Design review of the part built by this model. Coordinates are the model's own, in mm. Coordinates: 2 decimals unless noted, no trailing zeros. Order: outer loops, then holes, each group sorted by start corner. A loop starts at its lowest first (then second) coordinate and runs counter-clockwise, first axis right, second up. Notation, with made-up numbers: M 78,61.25 L 114,61.25 A25 cw 114,87.25 Z; hole C 87.25,3 d9. An arc over 180 degrees is marked long. Answer in a Markdown table with one row per item.
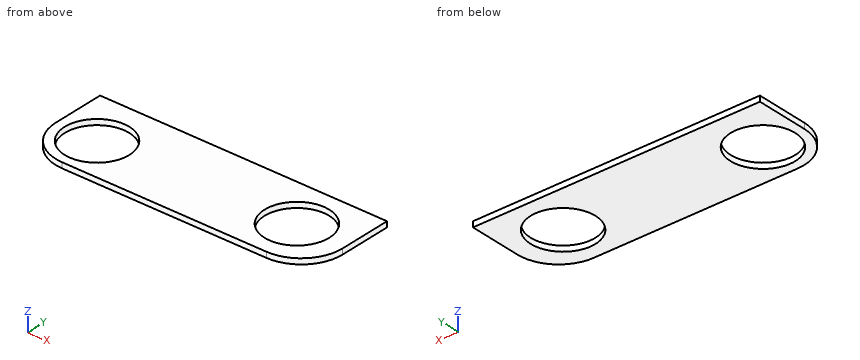
from build123d import *

# Parameters (mm, degrees)
SKETCH_R  = 58.5
PAD_DEPTH = 10


with BuildPart() as part:
    # Sketch → Pad (new body)
    with BuildSketch(Plane.XY):
        with BuildLine():
            Line((75, 0), (445, 0))
            ThreePointArc((445, 0), (498.033009, 21.966991), (520, 75))
            Line((520, 75), (520, 170))
            Line((520, 170), (0, 170))
            Line((0, 170), (0, 75))
            ThreePointArc((0, 75), (21.966991, 21.966991), (75, 0))
        make_face()
        with Locations((75, 74.82)):
            Circle(SKETCH_R, mode=Mode.SUBTRACT)
        with Locations((429.0695, 84.434)):
            Circle(SKETCH_R, mode=Mode.SUBTRACT)
    extrude(amount=PAD_DEPTH)


solid = part.part
(1) For line 1 along X through (y, z) = (56, 9.75); line 2 along X through (y, z) = (97.5, 4); line 3 along Y through (x, z) = (75, 7.75), list the stretches that pass through material, from the lowest coordinate up. Write a range as from..to.
Return value:
| item | result |
|---|---|
| line 1 | x = 2.45..19.61, 130.39..377.94, 480.19..517.55 |
| line 2 | x = 0..21.08, 128.92..372.05, 486.09..520 |
| line 3 | y = 0..16.32, 133.32..170 |
(2) Add section A-A, the plane y = 43. Give the boundary of the cut face in (x, z).
Return value:
| item | result |
|---|---|
| outline | M 7.17,0 L 25.91,0 L 25.91,10 L 7.17,10 Z; M 124.09,0 L 387.77,0 L 387.77,10 L 124.09,10 Z; M 470.37,0 L 512.83,0 L 512.83,10 L 470.37,10 Z |
(3) Insertion check: pin 1 Ø1 at (x, y) = (280.5, 90.5) entering from -Z. The pin has a flat end and moves straight along its axis. Give the tip position at first contact, or say it passes through.
Return value:
| item | result |
|---|---|
| pin 1 | stops at z = 0 |
(4) Add section C-C, the plane z = 4. Give the boundary of the cut face in (x, y), and give its area (3 significant figures).
Return value:
| item | result |
|---|---|
| outline | M 0,75 A75 ccw 75,0 L 445,0 A75 ccw 520,75 L 520,170 L 0,170 Z; hole C 75,74.82 d117; hole C 429.07,84.43 d117 |
| area | 64,500 mm2 |
(5) Add section D-D, the plane y = 111. Give the boundary of the cut face in (x, z), and give its area (3 significant figures).
Return value:
| item | result |
|---|---|
| outline | M 0,0 L 29.03,0 L 29.03,10 L 0,10 Z; M 120.97,0 L 376.95,0 L 376.95,10 L 120.97,10 Z; M 481.19,0 L 520,0 L 520,10 L 481.19,10 Z |
| area | 3,240 mm2 |
(6) Add section B-B, the plane x = 113.5. Give the boundary of the cut face in (y, z), and give its area (3 significant figures).
Return value:
| item | result |
|---|---|
| outline | M 0,0 L 30.77,0 L 30.77,10 L 0,10 Z; M 118.87,0 L 170,0 L 170,10 L 118.87,10 Z |
| area | 819 mm2 |
